from build123d import *

# Parameters (mm, degrees)
F1_DEPTH = 6
F2_R     = 6
F3_DEPTH = 25


with BuildPart() as f1:
    # F0 (on Top) → F1 (new body, symmetric)
    with BuildSketch(Plane.XY):
        with BuildLine():
            Line((-25.53717, 21.591896), (-24.523422, 17.280097))
            ThreePointArc((-24.523422, 17.280097), (-25.237606, 16.219225), (-25.905927, 15.128878))
            Line((-25.905927, 15.128878), (-30.249203, 14.259829))
            ThreePointArc((-30.249203, 14.259829), (-30.605918, 13.977255), (-30.585875, 13.52262))
            Line((-30.585875, 13.52262), (-28.398417, 9.671086))
            ThreePointArc((-28.398417, 9.671086), (-28.784789, 8.451977), (-29.118852, 7.217509))
            Line((-29.118852, 7.217509), (-33.041356, 5.16002))
            ThreePointArc((-33.041356, 5.16002), (-33.304011, 4.788394), (-33.156694, 4.357822))
            Line((-33.156694, 4.357822), (-29.972742, 1.27858))
            ThreePointArc((-29.972742, 1.27858), (-30, 0), (-29.972742, -1.27858))
            Line((-29.972742, -1.27858), (-33.156694, -4.357822))
            ThreePointArc((-33.156694, -4.357822), (-33.304011, -4.788394), (-33.041356, -5.16002))
            Line((-33.041356, -5.16002), (-29.118852, -7.217509))
            ThreePointArc((-29.118852, -7.217509), (-28.784789, -8.451977), (-28.398417, -9.671086))
            Line((-28.398417, -9.671086), (-30.585875, -13.52262))
            ThreePointArc((-30.585875, -13.52262), (-30.605918, -13.977255), (-30.249203, -14.259829))
            Line((-30.249203, -14.259829), (-25.905927, -15.128878))
            ThreePointArc((-25.905927, -15.128878), (-25.237606, -16.219225), (-24.523422, -17.280097))
            Line((-24.523422, -17.280097), (-25.53717, -21.591896))
            ThreePointArc((-25.53717, -21.591896), (-25.428316, -22.033761), (-25.00644, -22.204391))
            Line((-25.00644, -22.204391), (-20.594258, -21.814595))
            ThreePointArc((-20.594258, -21.814595), (-19.645822, -22.672487), (-18.661685, -23.489178))
            Line((-18.661685, -23.489178), (-18.419595, -27.911925))
            ThreePointArc((-18.419595, -27.911925), (-18.190663, -28.305223), (-17.737803, -28.350085))
            Line((-17.737803, -28.350085), (-13.614164, -26.733023))
            ThreePointArc((-13.614164, -26.733023), (-12.46245, -27.28896), (-11.28809, -27.795306))
            Line((-11.28809, -27.795306), (-9.809774, -31.970695))
            ThreePointArc((-9.809774, -31.970695), (-9.47931, -32.283565), (-9.032156, -32.199024))
            Line((-9.032156, -32.199024), (-5.531132, -29.485701))
            ThreePointArc((-5.531132, -29.485701), (-4.269445, -29.694643), (-3, -29.849623))
            Line((-3, -29.849623), (-0.405223, -33.43939))
            ThreePointArc((-0.405223, -33.43939), (0, -33.646484), (0.405223, -33.43939))
            Line((0.405223, -33.43939), (3, -29.849623))
            ThreePointArc((3, -29.849623), (4.269445, -29.694643), (5.531132, -29.485701))
            Line((5.531132, -29.485701), (9.032156, -32.199024))
            ThreePointArc((9.032156, -32.199024), (9.47931, -32.283565), (9.809774, -31.970695))
            Line((9.809774, -31.970695), (11.28809, -27.795306))
            ThreePointArc((11.28809, -27.795306), (12.46245, -27.28896), (13.614164, -26.733023))
            Line((13.614164, -26.733023), (17.737803, -28.350085))
            ThreePointArc((17.737803, -28.350085), (18.190663, -28.305223), (18.419595, -27.911925))
            Line((18.419595, -27.911925), (18.661685, -23.489178))
            ThreePointArc((18.661685, -23.489178), (19.645822, -22.672487), (20.594258, -21.814595))
            Line((20.594258, -21.814595), (25.00644, -22.204391))
            ThreePointArc((25.00644, -22.204391), (25.428316, -22.033761), (25.53717, -21.591896))
            Line((25.53717, -21.591896), (24.523422, -17.280097))
            ThreePointArc((24.523422, -17.280097), (25.237606, -16.219225), (25.905927, -15.128878))
            Line((25.905927, -15.128878), (30.249203, -14.259829))
            ThreePointArc((30.249203, -14.259829), (30.605918, -13.977255), (30.585875, -13.52262))
            Line((30.585875, -13.52262), (28.398417, -9.671086))
            ThreePointArc((28.398417, -9.671086), (28.784789, -8.451977), (29.118852, -7.217509))
            Line((29.118852, -7.217509), (33.041356, -5.16002))
            ThreePointArc((33.041356, -5.16002), (33.304011, -4.788394), (33.156694, -4.357822))
            Line((33.156694, -4.357822), (29.972742, -1.27858))
            ThreePointArc((29.972742, -1.27858), (30, 0), (29.972742, 1.27858))
            Line((29.972742, 1.27858), (33.156694, 4.357822))
            ThreePointArc((33.156694, 4.357822), (33.304011, 4.788394), (33.041356, 5.16002))
            Line((33.041356, 5.16002), (29.118852, 7.217509))
            ThreePointArc((29.118852, 7.217509), (28.784789, 8.451977), (28.398417, 9.671086))
            Line((28.398417, 9.671086), (30.585875, 13.52262))
            ThreePointArc((30.585875, 13.52262), (30.605918, 13.977255), (30.249203, 14.259829))
            Line((30.249203, 14.259829), (25.905927, 15.128878))
            ThreePointArc((25.905927, 15.128878), (25.237606, 16.219225), (24.523422, 17.280097))
            Line((24.523422, 17.280097), (25.53717, 21.591896))
            ThreePointArc((25.53717, 21.591896), (25.428316, 22.033761), (25.00644, 22.204391))
            Line((25.00644, 22.204391), (20.594258, 21.814595))
            ThreePointArc((20.594258, 21.814595), (19.645822, 22.672487), (18.661685, 23.489178))
            Line((18.661685, 23.489178), (18.419595, 27.911925))
            ThreePointArc((18.419595, 27.911925), (18.190663, 28.305223), (17.737803, 28.350085))
            Line((17.737803, 28.350085), (13.614164, 26.733023))
            ThreePointArc((13.614164, 26.733023), (12.46245, 27.28896), (11.28809, 27.795306))
            Line((11.28809, 27.795306), (9.809774, 31.970695))
            ThreePointArc((9.809774, 31.970695), (9.47931, 32.283565), (9.032156, 32.199024))
            Line((9.032156, 32.199024), (5.531132, 29.485701))
            ThreePointArc((5.531132, 29.485701), (4.269445, 29.694643), (3, 29.849623))
            Line((3, 29.849623), (0.405223, 33.43939))
            ThreePointArc((0.405223, 33.43939), (0, 33.646484), (-0.405223, 33.43939))
            Line((-0.405223, 33.43939), (-3, 29.849623))
            ThreePointArc((-3, 29.849623), (-4.269445, 29.694643), (-5.531132, 29.485701))
            Line((-5.531132, 29.485701), (-9.032156, 32.199024))
            ThreePointArc((-9.032156, 32.199024), (-9.47931, 32.283565), (-9.809774, 31.970695))
            Line((-9.809774, 31.970695), (-11.28809, 27.795306))
            ThreePointArc((-11.28809, 27.795306), (-12.46245, 27.28896), (-13.614164, 26.733023))
            Line((-13.614164, 26.733023), (-17.737803, 28.350085))
            ThreePointArc((-17.737803, 28.350085), (-18.190663, 28.305223), (-18.419595, 27.911925))
            Line((-18.419595, 27.911925), (-18.661685, 23.489178))
            ThreePointArc((-18.661685, 23.489178), (-19.645822, 22.672487), (-20.594258, 21.814595))
            Line((-20.594258, 21.814595), (-25.00644, 22.204391))
            ThreePointArc((-25.00644, 22.204391), (-25.428316, 22.033761), (-25.53717, 21.591896))
        make_face()
    extrude(amount=F1_DEPTH, both=True)

    # F2 (on face) → F3 (cut)
    with BuildSketch(Plane(origin=(0, 0, -6), x_dir=(1, 0, 0), z_dir=(0, 0, -1))):
        Circle(F2_R)
    extrude(amount=-F3_DEPTH, mode=Mode.SUBTRACT)


solid = f1.part
Geometry check sheet. Reference: the model listing, model coordinates, mm. A direction names the side the tool comes from. Round coordinates to 2 decimals unless told otherwise and drop trailing zeros. Loops run counter-clockwise (first coordinate to the right, second up) from the corner with the lowest first, then second, coordinate; pieces in that order, holes last.
Item 1: Gauge pin test, flat ends, axial feed: pin 1 (2 mm diameter, centred on y = -14.5, z = 3.5, fed in from -X); pin 2 (2 mm diameter, centred on x = 21.5, z = -2.5, fed in from -Y). Record the tip position at first contact, or that the pin passes through.
Item 2: Access from +Z, -Z, +X, -X, +Y, -Y to the whole of each face (thin tool, end or side, straight path). Record for faces 1 (the flat face through (15.7, 27.55, 0.08)), 2 (the flat face through (25.04, -19.47, 0.08)), 3 (the cylindrical face through (-12.48, -27.28, 0.08)), 4 (the flat face through (-25.023, -19.406, 0.084)).
Item 3: Cross-section at A-A on y = 0. Record the boundary of the cut face in (x, z).
Item 4: Mould release check, pull along X, two halves, no side actions. Record for faces 5 (the cylindrical face through (-30, 0, 0)), 6 (the flat face through (28.05, -14.7, 0.08)), 7 (the cylindrical face through (-4.29, -29.69, 0.08)): pulls with the +X half, pulls with the -X half, needs draft (parallel to the pull), parting line crosses it, or undercut.
Item 5: Cross-section at B-B on x = 22. Record the boundary of the cut face in (y, z).
Item 6: Cross-section at C-C on y = -16.5. Record the boundary of the cut face in (x, z), then the cut area to 3 significant figures.
Item 7: Thickness scan on line 1 (X direction, y = 0, z = 1.25); line 2 (Y direction, x = 0, z = -0.75); line 3 (X direction, y = -30, z = 2.5). Record the ranges inside material, lowest first.
Answer sheet:
1. pin 1: stops at x = -30.65
1. pin 2: stops at y = -21.98
2. face 1: +Z, -Z, +Y
2. face 2: +Z, -Z, +X
2. face 3: +Z, -Z, -Y
2. face 4: +Z, -Z, -X
3. outline: (-30, -6) - (-6, -6) - (-6, 6) - (-30, 6) - close; (6, -6) - (30, -6) - (30, 6) - (6, 6) - close
4. face 5: pulls with the -X half
4. face 6: pulls with the +X half
4. face 7: undercut
5. outline: (-21.94, -6) - (21.94, -6) - (21.94, 6) - (-21.94, 6) - close
6. outline: (-25.05, -6) - (25.05, -6) - (25.05, 6) - (-25.05, 6) - close
6. area: 601 mm2
7. line 1: x = -30 to -6, 6 to 30
7. line 2: y = -33.65 to -6, 6 to 33.65
7. line 3: x = -10.51 to -6.19, -2.89 to 2.89, 6.19 to 10.51
